Build history of the part. All positions in model axes, mm. Face numbers are marked on the shaded views. A direction names the side the tool comes from. Round coordinates to 2 decimals unless told otherwise and drop trailing zeros. Write each loop counter-clockwise with the first axis right and the second up, starting at its lowest first coordinate (ties: lowest second). Pieces come first, ordered by that corner, then holes. Notation, with made-up numbers: (63, 12) -> (113, 12) arc R27 ccw to (113, 38) -> close; hole circle Ø10 at (89, 57). An arc over 180 degrees is marked (long way). Answer in a Markdown table with one row per item. Add a question column.
from build123d import *

# Parameters (mm, degrees)
F0_R     = 4.953
F1_DEPTH = 4.7625
F2_DEPTH = 17.4625
F3_W     = 142.875
F3_H     = 25.654
F4_DEPTH = 3.175
F6_DEPTH = 4.7625
F8_DEPTH = 4.7625


with BuildPart() as f1:
    # F0 (on Top) → F1 (new body, symmetric)
    with BuildSketch(Plane.XY):
        with BuildLine():
            ThreePointArc((9.746036, 5.338768), (5.663947, 9.56072), (0, 11.1125))
            Line((0, 11.1125), (-14.2875, 11.1125))
            Line((-14.2875, 11.1125), (-14.2875, -11.1125))
            Line((-14.2875, -11.1125), (0, -11.1125))
            ThreePointArc((0, -11.1125), (9.56072, -5.663947), (9.746036, 5.338768))
        make_face()
        Circle(F0_R, mode=Mode.SUBTRACT)
    extrude(amount=F1_DEPTH, both=True)

    # F0 (on Top) → F2 (join, symmetric)
    with BuildSketch(Plane.XY):
        Polygon((-14.2875, -11.1125), (-14.2875, 11.1125), (-14.2875, 49.2125), (-14.2875, 131.7625), (-20.6375, 131.7625), (-20.6375, -11.1125), align=None)
    extrude(amount=F2_DEPTH, both=True)

    # F3 (on face) → F4 (cut)
    with BuildSketch(Plane(origin=(-20.6375, 0, 0), x_dir=(0, -1, 0), z_dir=(-1, 0, 0))):
        with Locations((-60.325, 0)):
            Rectangle(F3_W, F3_H)
    extrude(amount=-F4_DEPTH, mode=Mode.SUBTRACT)

    # F5 (on Top) → F8 (join, symmetric)
    with BuildSketch(Plane.XY):
        with BuildLine():
            Line((-14.2875, 11.1125), (0, 11.1125))
            ThreePointArc((0, 11.1125), (6.127987, 9.270136), (10.224032, 4.353943))
            Line((10.224032, 4.353943), (-14.2875, 61.9125))
            Line((-14.2875, 61.9125), (-14.2875, 11.1125))
        make_face()
    extrude(amount=F8_DEPTH, both=True)


with BuildPart() as f6:
    # F5 (on Top) → F6 (new body, symmetric)
    with BuildSketch(Plane.XY):
        with BuildLine():
            Line((-14.2875, 11.1125), (0, 11.1125))
            ThreePointArc((0, 11.1125), (6.127987, 9.270136), (10.224032, 4.353943))
            Line((10.224032, 4.353943), (-14.2875, 61.9125))
            Line((-14.2875, 61.9125), (-14.2875, 11.1125))
        make_face()
    extrude(amount=F6_DEPTH, both=True)


solid = f1.part
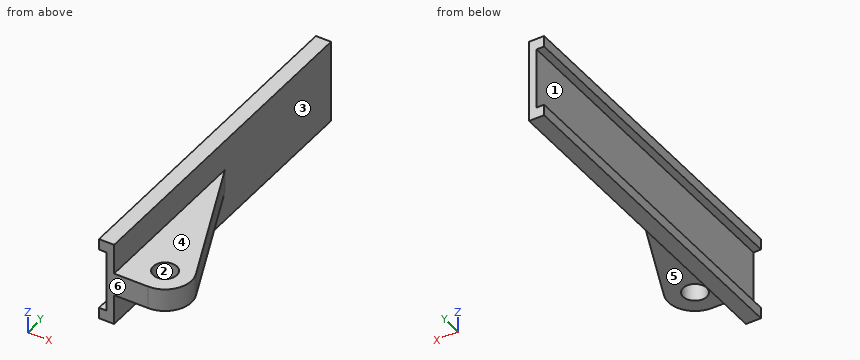
(1) Which spindle directions (+Z, -Z, +X, -X, +Y, -Y) get a long thin tool onto all of the face, cutting with end or side? Do the marked faces 5 and 6. Say none if no direction does.
(2) Saw through at B-B (y = 0). List the corners of the cut face in (x, z), plus the area to 3 significant figures.
(3) Saw through at A-A (z = -3). List the corners of the cut face in (x, y) (1 decimal).
(4) Probe line 1 along Z through (x, y) = (4.5, 9.5); line 2 along X through (y, z) = (78.5, -8.5); line 3 along Y through (x, z) = (0, 1). List the from-to ranges inside material, lowest first.
(5) Drop flat-ended pins along their axis: P1, Ø10, axis at y = 73.5, z = -2.5, coming from the -X side; P2, Ø13, axis at x = 0, y = 0, coming from the -Z side; P3, Ø10.5, axis at y = 74, z = 8, coming from the +X side. Give the stop position or say it passes through.
(6) Saw through at D-D (x = -10). List the corners of the cut face in (y, z), plus the area to 3 significant figures.
(7) Saw through at C-C (y = 94.5). List the corners of the cut face in (x, z), plus the area to 3 significant figures.
(8) Mould opens along X. For the marked faces 1, 2, 3 and 4 say: pulls with the +X half, pulls with the -X half, needs draft (parallel to the pull), parting line crosses it, or undercut.
Answer sheet:
| question | item | result |
|---|---|---|
| 1 | face 5 | -Z, +X, +Y, -Y |
| 1 | face 6 | +Z, -Z, +X, -X, -Y |
| 2 | outline | (-20.64, -17.46) -> (-14.29, -17.46) -> (-14.29, -4.76) -> (-4.95, -4.76) -> (-4.95, 4.76) -> (-14.29, 4.76) -> (-14.29, 17.46) -> (-20.64, 17.46) -> (-20.64, 12.83) -> (-17.46, 12.83) -> (-17.46, -12.83) -> (-20.64, -12.83) -> close; (4.95, -4.76) -> (11.11, -4.76) -> (11.11, 4.76) -> (4.95, 4.76) -> close |
| 2 | area | 288 mm² |
| 3 | outline | (-17.5, -11.1) -> (0, -11.1) arc R11.1 ccw to (10.2, 4.4) -> (-14.3, 61.9) -> (-14.3, 131.8) -> (-17.5, 131.8) -> close; hole circle Ø9.9 at (0, 0) |
| 4 | line 1 | z = -4.76 to 4.76 |
| 4 | line 2 | x = -17.46 to -14.29 |
| 4 | line 3 | y = -11.11 to -4.95, 4.95 to 28.36 |
| 5 | P1 | stops at x = -17.46 |
| 5 | P2 | stops at z = -4.76 |
| 5 | P3 | stops at x = -14.29 |
| 6 | outline | (-11.11, -4.76) -> (51.84, -4.76) -> (51.84, 4.76) -> (-11.11, 4.76) -> close |
| 6 | area | 600 mm² |
| 7 | outline | (-20.64, -17.46) -> (-14.29, -17.46) -> (-14.29, 17.46) -> (-20.64, 17.46) -> (-20.64, 12.83) -> (-17.46, 12.83) -> (-17.46, -12.83) -> (-20.64, -12.83) -> close |
| 7 | area | 140 mm² |
| 8 | face 1 | pulls with the -X half |
| 8 | face 2 | undercut |
| 8 | face 3 | pulls with the +X half |
| 8 | face 4 | needs draft |
